Build history of the part. All positions in model axes, mm. A direction names the side the tool comes from. Round coordinates to 2 decimals unless told otherwise and drop trailing zeros. Loops run counter-clockwise (first coordinate to the right, second up) from the corner with the lowest first, then second, coordinate; pieces in that order, holes last. Notation, with made-up numbers: (-24, 25.5) -> (-16, 25.5) arc R17 cw to (-16, 47.5) -> close; hole circle Ø5 at (77, 51). An arc over 180 degrees is marked (long way). Put each result on its own line as item: value. Start each with the question number.
Item 1: Cut at D-D, the plane y = 16. List the corners of the cut face in (x, z).
Item 2: Tool access for faces 1 (the cylindrical face through (-0.16, 11.9, 1.56)), 2 (the flat face through (7, 18, 0)), 3 (the flat face through (3.66, -12.4, 1)), 4 (the flat face through (-0.07, 15.54, 5.34)), 5 (the flat face through (-3.66, -12.4, -1.1)): list every direction of +Z, -Z, +X, -X, +Y, -Y with a clear straight run to the whole face (end or side of a thin tool).
Item 3: Cut at B-B, the plane y = 0. List the corners of the cut face in (x, z), plus the area to 3 significant figures.
Item 4: Cut at C-C, the plane z = 2. List the corners of the cut face in (x, y).
Item 5: Cut at A-A, the plane x = -1.5. List the corners of the cut face in (y, z), plus the area to 3 significant figures.
Item 6: Flat gauge pins, fed straight in: pin 1 Ø6 at (x, y) = (-5, -10.5) entering from -Z; pin 2 Ø3 at (y, z) = (6, -9.5) entering from -X; pin 3 Ø5.5 at (y, z) = (-10, 1.5) entering from -X. Where does each tip first touch, or does it go through?
Item 7: Pull direction Z, two halves, no side cores. Call faces 6 (the flat face through (4.34, 15.54, 0.08)), 7 (the flat face through (0.16, 11.92, 11.16)), 8 (the flat face through (9.628, 13.437, -0.174)), 9 (the flat face through (0, 13, 0)): +Z half, -Z half, draft (parallel to the pull), parting line (faces both ways), or undercut.
Item 8: Drill centre lines: probe 1 along Z at (x, y) = (-3, 0); probe 2 along Y at (x, z) = (7, 0); probe 3 along X at (y, z) = (14.5, -2). Where is each one in solid material? Low to high. Write a range as [from, to].
```python
from build123d import *

# Parameters (mm, degrees)
SKETCH_2_R               = 12
EXTRUDE_1_DEPTH          = 25
SKETCH_3_W               = 10
SKETCH_3_H               = 12
CUT_EXTRUDE_1_DEPTH      = 5
CUT_EXTRUDE_1_DRAFT      = -15
CUT_EXTRUDE_2_DEPTH      = 35.263683398
CUT_EXTRUDE_2_DEPTH_BACK = 35.263683398
SKETCH_4_OUTSIDE_W       = 65.4
SKETCH_4_OUTSIDE_H       = 48.4


with BuildPart() as part:
    # 草图2 → 凸台-拉伸1 (new, symmetric)
    with BuildSketch(Plane(origin=(0, 0, 0), x_dir=(0, 0, -1), z_dir=(1, 0, 0))):
        with BuildLine():
            Line((-13.743313889, 6.010101774), (-8.5, 18))
            Line((-8.5, 18), (8.5, 18))
            Line((8.5, 18), (13.743313889, 6.010101774))
            ThreePointArc((13.743313889, 6.010101774), (0, -15), (-13.743313889, 6.010101774))
        make_face()
        Circle(SKETCH_2_R, mode=Mode.SUBTRACT)
    extrude(amount=EXTRUDE_1_DEPTH, both=True)


with BuildPart() as cut_extrude_1_tool:
    # 草图3 → 切除-拉伸1 (with draft: the straight prism first)
    with BuildSketch(Plane(origin=(0, 18, 0), x_dir=(1, 0, 0), z_dir=(0, 1, 0))):
        Rectangle(SKETCH_3_W, SKETCH_3_H)
    extrude(amount=-CUT_EXTRUDE_1_DEPTH)
    # 切除-拉伸1: the draft: its side faces are tilted about the plane it starts from
    cut_extrude_1_sides = [cut_extrude_1_tool.faces().sort_by_distance(p)[0] for p in [
        (-5, 15.5, 0),
        (0, 15.5, 6),
        (5, 15.5, 0),
        (0, 15.5, -6),
    ]]
    draft(cut_extrude_1_sides, Plane(origin=(0, 18, 0), x_dir=(1, 0, 0), z_dir=(0, 1, 0)), CUT_EXTRUDE_1_DRAFT)


with BuildPart() as part_1:
    add(part.part)

    # 切除-拉伸1: cut by cut_extrude_1_tool
    add(cut_extrude_1_tool.part, mode=Mode.SUBTRACT)

    # 草图4 outside → 切除-拉伸2 (cut, two sides: drawn at the far end of the back side and taken through both)
    with BuildSketch(Plane.XY.offset(-CUT_EXTRUDE_2_DEPTH_BACK)):
        with Locations((0, 1.5)):
            Rectangle(SKETCH_4_OUTSIDE_W, SKETCH_4_OUTSIDE_H)
        with BuildLine():
            Line((7.5, 18), (-7.5, 18))
            Line((-7.5, 18), (-11.696768923, 9))
            ThreePointArc((-11.696768923, 9), (-5.825685936, 3.477922356), (-3.660254038, -4.285701903))
            Line((-3.660254038, -4.285701903), (-3.660254038, -15))
            Line((-3.660254038, -15), (3.660254038, -15))
            Line((3.660254038, -15), (3.660254038, -4.285701903))
            ThreePointArc((3.660254038, -4.285701903), (5.825685936, 3.477922356), (11.696768923, 9))
            Line((11.696768923, 9), (7.5, 18))
        make_face(mode=Mode.SUBTRACT)
    extrude(amount=CUT_EXTRUDE_2_DEPTH + CUT_EXTRUDE_2_DEPTH_BACK, mode=Mode.SUBTRACT)


solid = part_1.part
```
Reply:
1. outline: (-8.43, -9.37) -> (8.43, -9.37) -> (8.43, 9.37) -> (-8.43, 9.37) -> close; hole (-4.46, -5.46) -> (4.46, -5.46) -> (4.46, 5.46) -> (-4.46, 5.46) -> close
2. face 1: +X, -X
2. face 2: +Z, -Z, +X, -X, +Y
2. face 3: +Z, -Z, +X, -Y
2. face 4: +Y
2. face 5: +Z, -Z, -X, -Y
3. outline: (-4.29, -15) -> (4.29, -15) -> (4.29, -12) -> (-4.29, -12) -> close; (-4.29, 12) -> (4.29, 12) -> (4.29, 15) -> (-4.29, 15) -> close
3. area: 51.4 mm^2
4. outline: (-10.38, 11.83) -> (10.38, 11.83) -> (7.5, 18) -> (5, 18) -> (3.66, 13) -> (-3.66, 13) -> (-5, 18) -> (-7.5, 18) -> close; (-3.66, -14.87) -> (3.66, -14.87) -> (3.66, -11.83) -> (-3.66, -11.83) -> close
5. outline: (6.01, -13.74) -> (18, -8.5) -> (18, -6) -> (13, -4.66) -> (13, 4.66) -> (18, 6) -> (18, 8.5) -> (6.01, 13.74) arc R15 ccw (long way) to start; hole circle Ø24 at (0, 0)
5. area: 290 mm^2
6. pin 1: stops at z = -12.8
6. pin 2: stops at x = -9.38
6. pin 3: stops at x = -3.66
7. face 6: undercut
7. face 7: +Z half
7. face 8: draft
7. face 9: undercut
8. probe 1: z = [-15, -12], [12, 15]
8. probe 2: y = [12, 18]
8. probe 3: x = [-9.13, -4.06], [4.06, 9.13]
